Autodesk Inventor part; units mm, degrees
ref_plane "YZ Plane" through (0, 0, 0) normal (1, 0, 0) x (0, 1, 0)
ref_plane "XZ Plane" through (0, 0, 0) normal (0, 1, 0) x (-1, 0, 0)
ref_plane "XY Plane" through (0, 0, 0) normal (0, 0, 1) x (1, 0, 0)
sketch "Sketch1" plane through (0, 0, 0) normal (0, 0, 1) x (1, 0, 0)
  circle A0 centre (0, 0) radius 3.175
  dimension "d0" = 6.35
extrude "Extrusion1" add sketch "Sketch1" along normal blind 11.5824
hole "Hole1" at (0, 0, 0) direction (0, 0, 1) diameter 4.9784 end through all
sketch "Sketch2" plane through (0, 0, 11.5824) normal (0, 0, 1) x (1, 0, 0)
  circle A0 centre (0, 0) radius 3.175
  circle A1 centre (0, 0) radius 3.9688
  dimension "d10" = 7.9375
extrude "Extrusion2" add sketch "Sketch2" against normal blind 1.6256
properties part number "Tensioning Shaft"
The listing builds one solid part. Answer for the finished solid, in the listing's coordinates (mm). A direction names the side the tool comes from. Coordinates: 2 decimals unless noted, no trailing zeros. Order: outer loops, then holes, each group sorted by start corner. A loop starts at its lowest first (then second) coordinate and runs counter-clockwise, first axis right, second up. Notation, with made-up numbers: (87.25, 51) -> (98.25, 51) arc R22 ccw to (98.25, 87) -> close; hole circle Ø1 at (47.25, 1.5). An arc over 180 degrees is marked (long way). Answer in a Markdown table with one row per item. Add a question column.
Item 1: Each of these flat-tipped pins is pushed along its axis until it touches: P1, Ø1, axis at x = 3, y = 2.5, coming from the -Z side; P2, Ø3, axis at y = 2, z = 5, coming from the -X side; P3, Ø4, axis at y = 0, z = 2, coming from the -X side (3 decimals). Where does it stop, or does it pass through?
Item 2: Find section D-D (y = -2.75). Write down the section's boundary in (x, z).
Item 3: Which of the six approach directions +Z, -Z, +X, -X, +Y, -Y give full straight-line access (tool end or side, diameter ignored) to faces 1 (the face through (3.666, -1.52, 10.781)), 2 (the face through (-2, 3, 9.957))?
Item 4: Find section A-A (x = 0). Write down the section's boundary in (y, z) (3 decimals).
Item 5: Find section C-C (z = 2.25). Write down the section's boundary in (x, y) (3 decimals), then the cut area to 3 significant figures.
Item 6: Determine the mould class of faces 3 (the face through (-0.748, 2.374, 5.872)), 4 (the face through (-0.69, 3.1, 4.91)), 5 (the face through (2, 2, 11.582)) for opening direction X: +X half, -X half, draft (parallel to the pull), parting line (faces both ways), or undercut.
Item 7: Find the intervals of material crossed by L1, parallel to Y at x = 0, z = 8.5 (3 decimals); L2, parallel to Y at x = -0.5, z = 5.5; L3, parallel to X at y = 1.25, z = 10.75, in increasing order. Write a range as from..to.
Result set:
| question | item | result |
|---|---|---|
| 1 | P1 | stops at z = 9.96 |
| 1 | P2 | stops at x = -3.14 |
| 1 | P3 | stops at x = -3.175 |
| 2 | outline | (-2.86, 9.96) -> (-1.59, 9.96) -> (-1.59, 0) -> (1.59, 0) -> (1.59, 9.96) -> (2.86, 9.96) -> (2.86, 11.58) -> (-2.86, 11.58) -> close |
| 3 | face 1 | +Z, -Z |
| 3 | face 2 | -Z |
| 4 | outline | (-3.969, 9.957) -> (-3.175, 9.957) -> (-3.175, 0) -> (-2.489, 0) -> (-2.489, 11.582) -> (-3.969, 11.582) -> close; (2.489, 0) -> (3.175, 0) -> (3.175, 9.957) -> (3.969, 9.957) -> (3.969, 11.582) -> (2.489, 11.582) -> close |
| 5 | outline | circle Ø6.35 at (0, 0); hole circle Ø4.978 at (0, 0) |
| 5 | area | 12.2 mm² |
| 6 | face 3 | undercut |
| 6 | face 4 | parting line |
| 6 | face 5 | draft |
| 7 | L1 | y = -3.175..-2.489, 2.489..3.175 |
| 7 | L2 | y = -3.14..-2.44, 2.44..3.14 |
| 7 | L3 | x = -3.77..-2.15, 2.15..3.77 |
